```python
from build123d import *

# Parameters (mm, degrees)
SKETCH_1_W      = 13
SKETCH_1_H      = 10
EXTRUDE_1_DEPTH = 8
SKETCH_2_R      = 3
EXTRUDE_2_DEPTH = 9
SKETCH_6_R      = 1.5
EXTRUDE_3_DEPTH = 11
EXTRUDE_3_TAPER = 1
FILLET_1_R      = 0.5
SKETCH_7_W      = 0.6
SKETCH_7_H      = 2.6
EXTRUDE_4_DEPTH = 5


with BuildPart() as part:
    # 草图1 → 凸台-拉伸1 (new body)
    with BuildSketch(Plane(origin=(0, 0, 0), x_dir=(1, 0, 0), z_dir=(0, 1, 0))):
        Rectangle(SKETCH_1_W, SKETCH_1_H)
    extrude(amount=EXTRUDE_1_DEPTH)

    # 草图2 → 凸台-拉伸2 (add)
    with BuildSketch(Plane(origin=(0, 8, 0), x_dir=(1, 0, 0), z_dir=(0, 1, 0))):
        with Locations(Location((0, 0, 0), (0, 0, 270))):
            Circle(SKETCH_2_R)
    extrude(amount=EXTRUDE_2_DEPTH)

    # 草图6 → 凸台-拉伸3 (add)
    with BuildSketch(Plane(origin=(0, 17, 0), x_dir=(1, 0, 0), z_dir=(0, 1, 0))):
        Circle(SKETCH_6_R)
    extrude(amount=EXTRUDE_3_DEPTH, taper=EXTRUDE_3_TAPER)

    # 圆角1
    fillet_1_edges = [part.edges().sort_by_distance(p)[0] for p in [
        (-1.307994286, 28, 0),
    ]]
    fillet(fillet_1_edges, radius=FILLET_1_R)

    # 草图7 → 凸台-拉伸4 (add)
    with BuildSketch(Plane.XZ):
        with Locations((-4.6, 0)):
            Rectangle(SKETCH_7_W, SKETCH_7_H)
        Rectangle(SKETCH_7_W, SKETCH_7_H)
        with Locations((4.6, -0.156510549)):
            Rectangle(SKETCH_7_W, SKETCH_7_H)
    extrude(amount=EXTRUDE_4_DEPTH)


solid = part.part
```
Read the model definition and answer for the solid it produces. Units are mm, in the model's axes. A direction names the side the tool comes from. Coordinates: 2 decimals unless noted, no trailing zeros. Write each loop counter-clockwise with the first axis right and the second up, starting at its lowest first coordinate (ties: lowest second). Pieces come first, ordered by that corner, then holes. Notation, with made-up numbers: (-13.75, 12.25) -> (-0.75, 12.25) arc R25 ccw to (-0.75, 39.25) -> close; hole circle Ø11 at (-14, 61.5). An arc over 180 degrees is marked (long way). Answer as a JSON object with one key per item and string values.
Q1. Determine the mould class of faces 1 (the flat face through (4.3, -2, 0)), 2 (the cylindrical face through (0.9, 12.44, 2.86)), 3 (the flat face through (0, 4, -5)) for opening direction X: pulls with the +X half, pulls with the -X half, needs draft (parallel to the pull), parting line crosses it, or undercut.
The answers:
{"face 1": "undercut", "face 2": "parting line crosses it", "face 3": "needs draft"}
Q2. The part is cut by section A-A on y = -1. Give the vertices of the cut face in (x, z).
The answers:
{"outline": "(-4.9, -1.3) -> (-4.3, -1.3) -> (-4.3, 1.3) -> (-4.9, 1.3) -> close; (-0.3, -1.3) -> (0.3, -1.3) -> (0.3, 1.3) -> (-0.3, 1.3) -> close; (4.3, -1.46) -> (4.9, -1.46) -> (4.9, 1.14) -> (4.3, 1.14) -> close"}
Q3. The part is cut by section C-C on x = -5.25. Give the vertices of the cut face in (y, z), then the cut area to 3 significant figures.
The answers:
{"outline": "(0, -5) -> (8, -5) -> (8, 5) -> (0, 5) -> close", "area": "80.0 mm2"}
Q4. Flat-ended cylindrical pins translate along their axes: pin 1 Ø0.7 at (x, y) = (4.5, -2) entering from +Z; pin 2 Ø5 at (x, y) = (5, 20) entering from +Z; pin 3 Ø0.5 at (x, y) = (4.5, -3) entering from -Z; pin 4 Ø4 at (y, z) = (20, -2) entering from +X. Find the tip coordinate at first contact, or state that the pin passes through.
The answers:
{"pin 1": "stops at z = 1.14", "pin 2": "passes through", "pin 3": "stops at z = -1.46", "pin 4": "stops at x = 1.46"}
Q5. Consider line 1 (Y direction, x = 4.75, z = -4.5); line 2 (Y direction, x = -0.25, z = 2); line 3 (X direction, y = 16, z = 0.5). Determine where each line is inside the solid, lowest interval first. Write a range as [from, to].
The answers:
{"line 1": "y = [0, 8]", "line 2": "y = [0, 17]", "line 3": "x = [-2.96, 2.96]"}
Q6. The part is cut by section B-B on z = -2.5. Give the vertices of the cut face in (x, y).
The answers:
{"outline": "(-6.5, 0) -> (6.5, 0) -> (6.5, 8) -> (1.66, 8) -> (1.66, 17) -> (-1.66, 17) -> (-1.66, 8) -> (-6.5, 8) -> close"}
Q7. The part is cut by section D-D on y = 11. Give the vertices of the cut face in (x, z).
The answers:
{"outline": "circle Ø6 at (0, 0)"}
Q8. A tool of negligible diameter and unlimited length cuts with its end or side. For faces 4 (the conical face through (-0.183, 22.328, -1.395)), 5 (the flat face through (-4.9, -2, 0)), 6 (the flat face through (-4.3, -2, 0)), 7 (the flat face through (4.9, -2, 0)), from which of +Z, -Z, +X, -X, +Y, -Y can it reach the whole face along a straight path? Write none if from no direction.
The answers:
{"face 4": "+Y", "face 5": "+Z, -Z, -X, -Y", "face 6": "+Z, -Z, -Y", "face 7": "+Z, -Z, +X, -Y"}
